from build123d import *

# Parameters (mm, degrees)
F1_DEPTH = 5
F2_SIZE2 = 5.958758
F2_SIZE  = 4.99999
F4_R     = 4.75
F5_DEPTH = 30
F7_DEPTH = 6
F8_SIZE2 = 3
F8_SIZE  = 3


# Not quite as in the source:
# - a fillet or chamfer is up to 0.001 mm smaller than in the source, because OpenCascade refuses the exact size


with BuildPart() as f1:
    # F0 (on Top) → F1 (new body)
    with BuildSketch(Plane.XY):
        Polygon((-12.0511064306, 53.3692054451), (-12.0511064306, -68.6175450683), (12.0511064306, -68.6175450683), (12.0511064306, 53.3692054451), (0, 68.6175450683), align=None)
        Polygon((12.0511064306, -68.6175450683), (-12.0511064306, -68.6175450683), (-28.6420956254, -68.6175450683), (-6.6773975268, -75.6341889501), (6.4345644787, -75.6341889501), (28.3992625773, -68.6175450683), align=None)
    extrude(amount=F1_DEPTH)

    # F2 (size 5 and 5.958767963 in the source; OpenCascade refuses exactly that, so slightly less here)
    f2_edges = [f1.edges().sort_by_distance(p)[0] for p in [
        (12.051106, -7.62417, 5),
        (6.025553, 60.993375, 5),
        (-6.025553, 60.993375, 5),
        (-12.051106, -7.62417, 5),
    ]]
    chamfer(f2_edges, length=F2_SIZE, length2=F2_SIZE2)

    # F3: F1 across plane


with BuildPart() as f1_1:
    add(f1.part)
    add(f1.part.mirror(Plane.XY))

    # F4 (on face) → F5 (join)
    with BuildSketch(Plane.XZ.offset(75.6341889501)):
        Circle(F4_R)
    extrude(amount=F5_DEPTH)

    # F6 (on face) → F7 (join)
    with BuildSketch(Plane.XZ.offset(105.6341889501)):
        Polygon((3.3913787161, 1.6732233375), (0, 3.7816829499), (-3.2607477523, 1.9153720341), (-3.2607477523, -1.9153720341), (0, -3.7816829499), (3.3913787161, -1.6732233375), align=None)
    extrude(amount=F7_DEPTH)

    # F8
    f8_edges = [f1_1.edges().sort_by_distance(p)[0] for p in [
        (-1.630374, -111.634189, 2.848527),
        (1.695689, -111.634189, 2.727453),
        (-3.260748, -111.634189, 0),
        (-1.630374, -111.634189, -2.848527),
        (1.695689, -111.634189, -2.727453),
        (3.391379, -111.634189, 0),
    ]]
    chamfer(f8_edges, length=F8_SIZE, length2=F8_SIZE2)


solid = f1_1.part
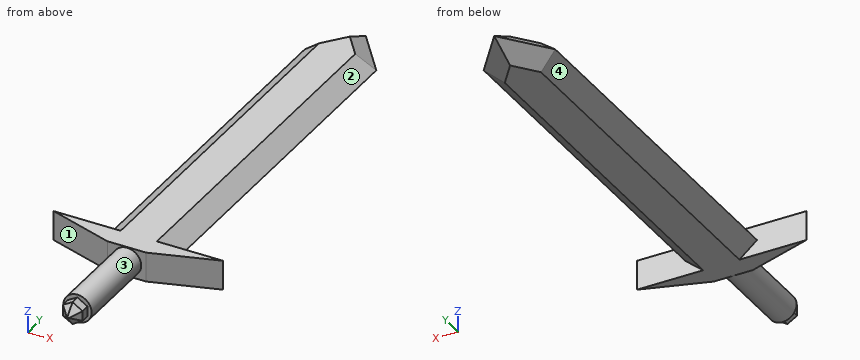
For this review, take the finished solid that the model builds, in its own axes (mm). Face numbers are marked on the shaded views. A direction names the side the tool comes from. Round coordinates to 2 decimals unless told otherwise and drop trailing zeros. Order: outer loops, then holes, each group sorted by start corner. A loop starts at its lowest first (then second) coordinate and runs counter-clockwise, first axis right, second up. Notation, with made-up numbers: M 56,-23.75 L 62,-23.75 A27 ccw 62,2.25 Z; hole C 0,51 d8. An arc over 180 degrees is marked long. Use a Markdown table: item, result. Add a question column.
Item 1: To check wall thickness, follow line 1 along X through (y, z) = (32, -1.5); line 2 along Y through (x, z) = (15, -1.75). State the ranges of each line that lie inside material, in increasing order.
Item 2: Add section B-B, the plane x = -18.5. Give the boundary of the cut face in (y, z), then the cut area to 3 significant figures.
Item 3: Add section A-A, the plane y = 29.5. Give the boundary of the cut face in (x, z).
Item 4: Tool access review of the marked faces 1, 2, 3 and 4: name each direction out of +Z, -Z, +X, -X, +Y, -Y from which nothing blocks a thin tool from reaching the whole face with its end or side.
Item 5: Insertion check: pin 1 (3 mm diameter, centred on x = 20, z = 2, fed in from +Y); pin 2 (2 mm diameter, centred on x = -10, y = -56, fed in from +Z); pin 3 (5 mm diameter, centred on x = -7, y = 36.5, fed in from -Z); pin 4 (3 mm diameter, centred on x = -12, z = -0.5, fed in from +Y). Each pin has a flat end and moves straight along its axis. Give the tip position at first contact, or say it passes through.
Geometry results:
| question | item | result |
|---|---|---|
| 1 | line 1 | x = -10.26 to 10.26 |
| 1 | line 2 | y = -72.9 to -68.62 |
| 2 | outline | M -71.86,-5 L -68.62,-5 L -68.62,5 L -71.86,5 Z |
| 2 | area | 32.4 mm² |
| 3 | outline | M -12.05,0 L -6.09,-5 L 6.09,-5 L 12.05,0 L 6.09,5 L -6.09,5 Z |
| 4 | face 1 | +Z, -Z, -X, -Y |
| 4 | face 2 | +Z, +X, +Y |
| 4 | face 3 | -Y |
| 4 | face 4 | -Z, -X, +Y |
| 5 | pin 1 | stops at y = -68.62 |
| 5 | pin 2 | stops at z = 2.56 |
| 5 | pin 3 | stops at z = -5 |
| 5 | pin 4 | stops at y = 55.22 |
